from build123d import *

# Parameters (mm, degrees)
BOX002_W     = 10
BOX002_H     = 10
BOX002_DEPTH = 10


with BuildPart() as cubo002:
    # Box002 → Box002 (new body)
    with BuildSketch(Plane(origin=(-5, -5, 0), x_dir=(1, 0, 0), z_dir=(0, 0, 1))):
        with Locations((5, 5)):
            Rectangle(BOX002_W, BOX002_H)
    extrude(amount=BOX002_DEPTH)


with BuildPart() as cut:
    # Sphere → Sphere (revolve)
    with BuildSketch(Plane.XZ):
        with BuildLine():
            ThreePointArc((0, -5), (5, 0), (0, 5))
            Line((0, 5), (0, -5))
        make_face()
    revolve(axis=Axis((0, 0, 0), (0, 0, 1)))

    # Cut: cut Cubo002
    add(cubo002.part, mode=Mode.SUBTRACT)


with BuildPart() as cut_1:
    # Cut placement: moved
    add(cut.part.moved(Location((-36, -35, -68))))


solid = cut_1.part
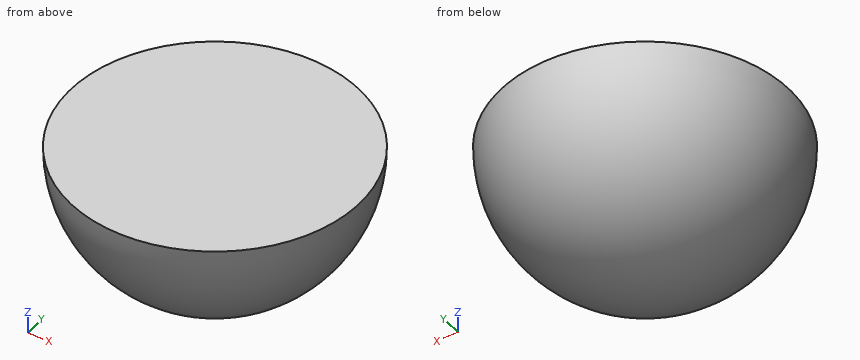
Design review of the part built by this model. Coordinates are the model's own, in mm. Coordinates: 2 decimals unless noted, no trailing zeros. Order: outer loops, then holes, each group sorted by start corner. A loop starts at its lowest first (then second) coordinate and runs counter-clockwise, first axis right, second up. Notation, with made-up numbers: (-38.75, 15) - (-1.75, 15) arc R35 cw to (-1.75, 51) - close; hole circle Ø2 at (-6, -27). An arc over 180 degrees is marked (long way). Put each result on its own line as item: value.
1) Take a section at B-B, the plane y = -38. Give the boundary of the cut face in (x, z).
Response values:
outline: (-40, -68) arc R4 ccw to (-32, -68) - close
2) Take a section at C-C, the plane z = -69.1. Give the boundary of the cut face in (x, y) (1 decimal), and give its area (3 significant figures).
Response values:
outline: circle Ø9.8 at (-36, -35)
area: 74.7 mm²
3) Take a section at D-D, the plane z = -71.2. Give the boundary of the cut face in (x, y).
Response values:
outline: circle Ø7.68 at (-36, -35)
4) Insertion check: P1, Ø1, axis at y = -39, z = -70.5, coming from the -X side; P2, Ø1, axis at x = -39.5, y = -36, coming from the -Z side; P3, Ø1, axis at y = -34.5, z = -71.5, coming from the -X side. Each pin has a flat end and moves straight along its axis. Give the tip position at first contact, or say it passes through.
Response values:
P1: stops at x = -38.69
P2: stops at z = -71.89
P3: stops at x = -39.97
5) Wall thickness on L1, parallel to Z at x = -38.5, y = -36; L2, parallel to X at y = -35.25, z = -71.2; L3, parallel to Z at x = -32.5, y = -34: over which ranges is each line inside the solid? List them lowest first. Write a range as from..to.
Response values:
L1: z = -72.21..-68
L2: x = -39.83..-32.17
L3: z = -71.43..-68
6) Take a section at A-A, the plane x = -39. Give the boundary of the cut face in (y, z).
Response values:
outline: (-39, -68) arc R4 ccw to (-31, -68) - close
